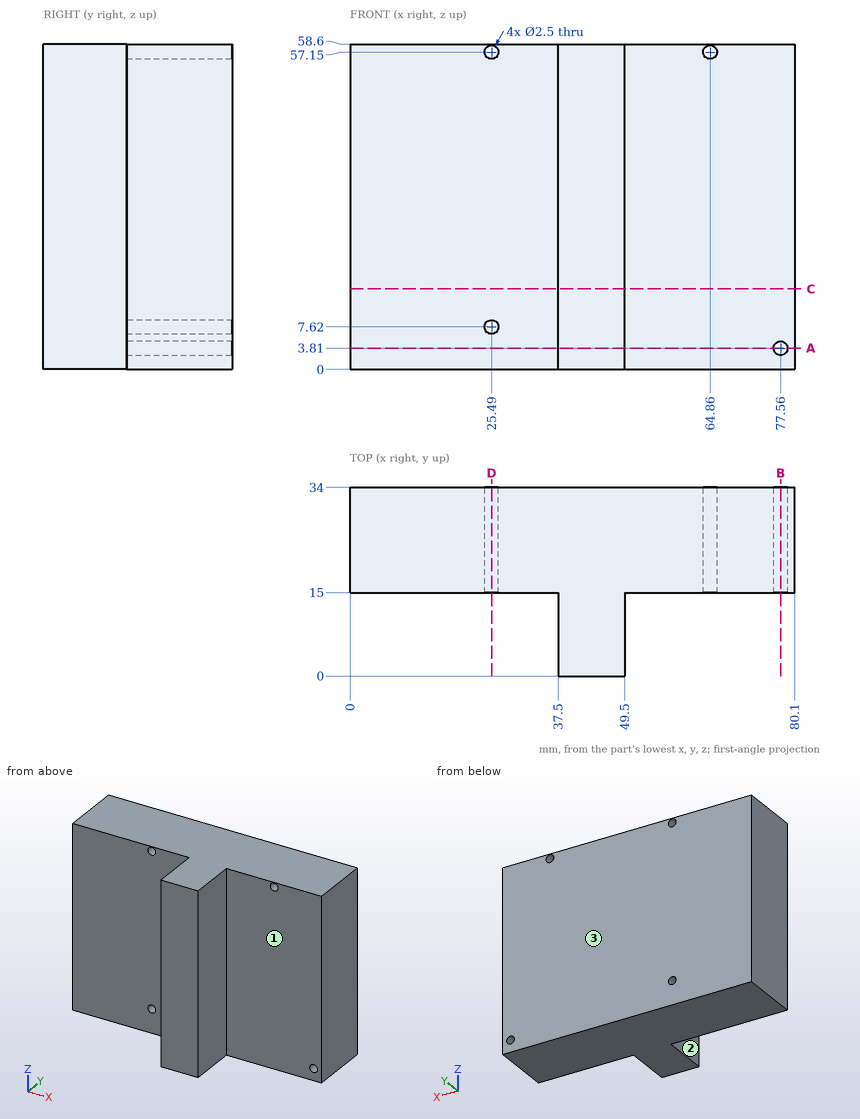
Job drawing, mm, ordinate dimensions from the low corner. One solid piece. A direction names the side the tool comes from. Coordinates: 2 decimals unless noted, no trailing zeros. Order: outer loops, then holes, each group sorted by start corner. A loop starts at its lowest first (then second) coordinate and runs counter-clockwise, first axis right, second up. Notation, with made-up numbers: (32, 19) -> (57, 19) arc R31 cw to (57, 50) -> close; hole circle Ø11 at (-39.5, 10.25). An arc over 180 degrees is marked (long way). Put each result on its own line as item: value. Start each with the question number.
(1) Which spindle directions (+Z, -Z, +X, -X, +Y, -Y) get a long thin tool onto all of the face, cutting with end or side? Do the marked faces 1, 2 and 3. Say none if no direction does.
(2) Pin check, flat tips, straight feed: pin 1 Ø12 at (y, z) = (9.5, 20.5) entering from -X; pin 2 Ø4 at (x, z) = (64.86, 57.15) entering from -Y; pin 3 Ø7.5 at (y, z) = (10, 21.5) entering from +X. Stop position of each tip, or through.
(3) Probe line 1 along X through (y, z) = (25.5, 57.15); line 2 along Y through (x, z) = (71, 39); line 3 along Z through (x, y) = (64.86, 30.25). List the from-to ranges inside material, lowest first. Write a range as [from, to].
(4) Band-saw the part on B-B (x = 77.56). Give the cut face in (y, z).
(5) Band-saw the part on A-A (z = 3.81). Give the cut face in (x, y), then the cut area to 3 significant figures.
(6) Band-saw the part on C-C (z = 14.5). Give the cut face in (x, y), then the cut area to 3 significant figures.
(7) Band-saw the part on D-D (x = 25.49). Give the cut face in (y, z).
Determined:
1. face 1: +Z, -Z, +X, -Y
1. face 2: +Z, -Z, -X, -Y
1. face 3: +Z, -Z, +X, -X, +Y
2. pin 1: stops at x = 0
2. pin 2: stops at y = 15
2. pin 3: stops at x = 49.5
3. line 1: x = [0, 24.24], [26.74, 63.61], [66.11, 80.1]
3. line 2: y = [15, 34]
3. line 3: z = [0, 55.9], [58.4, 58.6]
4. outline: (15, 0) -> (34, 0) -> (34, 2.56) -> (15, 2.56) -> close; (15, 5.06) -> (34, 5.06) -> (34, 58.6) -> (15, 58.6) -> close
5. outline: (0, 15) -> (37.5, 15) -> (37.5, 0) -> (49.5, 0) -> (49.5, 15) -> (76.31, 15) -> (76.31, 34) -> (0, 34) -> close; (78.81, 15) -> (80.1, 15) -> (80.1, 34) -> (78.81, 34) -> close
5. area: 1,650 mm²
6. outline: (0, 15) -> (37.5, 15) -> (37.5, 0) -> (49.5, 0) -> (49.5, 15) -> (80.1, 15) -> (80.1, 34) -> (0, 34) -> close
6. area: 1,700 mm²
7. outline: (15, 0) -> (34, 0) -> (34, 6.37) -> (15, 6.37) -> close; (15, 8.87) -> (34, 8.87) -> (34, 55.9) -> (15, 55.9) -> close; (15, 58.4) -> (34, 58.4) -> (34, 58.6) -> (15, 58.6) -> close
